Design review of the part shown in the three views and the two pictorial views. Dimensions are in mm from the part's minimum x, y and z. Give positions to 0.01 mm unless a question says otherwise; leave off trailing zeros. Order: outer loops, then holes, each group sorted by start corner. A loop starts at its lowest first (then second) coordinate and runs counter-clockwise, first axis right, second up.
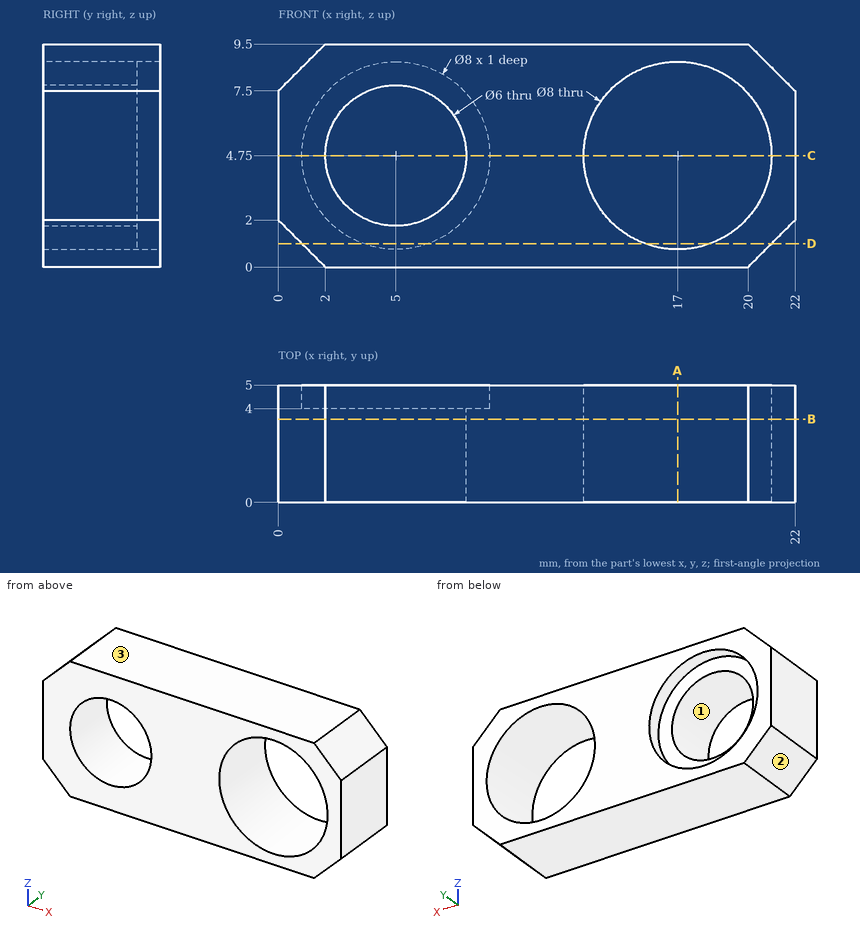
Item 1: Take a section at A-A (x = 17). Give the boundary of the cut face in (y, z).
Values found:
outline: (0, 0) - (5, 0) - (5, 0.75) - (0, 0.75) - close; (0, 8.75) - (5, 8.75) - (5, 9.5) - (0, 9.5) - close
Item 2: Take a section at C-C (z = 4.75). Give the boundary of the cut face in (x, y), and give its area (3 significant figures).
Values found:
outline: (0, 0) - (2, 0) - (2, 4) - (1, 4) - (1, 5) - (0, 5) - close; (8, 0) - (13, 0) - (13, 5) - (9, 5) - (9, 4) - (8, 4) - close; (21, 0) - (22, 0) - (22, 5) - (21, 5) - close
area: 38.0 mm2
Item 3: Draft analysis for pull direction X (two halves, no side actions). For the marked faces 1, 2 and 3, state which applies: released by +X, released by -X, zero draft, split by the parting line, or undercut.
Values found:
face 1: undercut
face 2: released by -X
face 3: zero draft
Item 4: Take a section at B-B (y = 3.55). Give the boundary of the cut face in (x, z).
Values found:
outline: (0, 2) - (2, 0) - (20, 0) - (22, 2) - (22, 7.5) - (20, 9.5) - (2, 9.5) - (0, 7.5) - close; hole circle Ø6 at (5, 4.75); hole circle Ø8 at (17, 4.75)
Item 5: Take a section at D-D (z = 1). Give the boundary of the cut face in (x, y), and give its area (3 significant figures).
Values found:
outline: (1, 0) - (15.61, 0) - (15.61, 5) - (6.39, 5) - (6.39, 4) - (3.61, 4) - (3.61, 5) - (1, 5) - close; (18.39, 0) - (21, 0) - (21, 5) - (18.39, 5) - close
area: 83.3 mm2
Item 6: Clearance check with flat-ended pins moving along their axes: pin 1 Ø1.5 at (x, z) = (14.5, 7) entering from -Y; pin 2 Ø5 at (x, z) = (5, 4.75) entering from +Y. State where each tip first meets the part, or that it passes through.
Values found:
pin 1: stops at y = 0
pin 2: passes through
Item 7: For line 1 (X direction, y = 4.25, z = 4.75); line 2 (X direction, y = 1.3, z = 4); line 3 (Z direction, x = 7.5, y = 2.55), list the stretches that pass through material, from the lowest coordinate up.
Values found:
line 1: x = 0 to 1, 9 to 13, 21 to 22
line 2: x = 0 to 2.1, 7.9 to 13.07, 20.93 to 22
line 3: z = 0 to 3.09, 6.41 to 9.5
